Could you check a few things on this drawing? It's one solid part, dimensions in mm from its lowest x, y, z. Give positions to 0.01 mm unless a question says otherwise; leave off trailing zeros. Use one line per item in the form item = value.
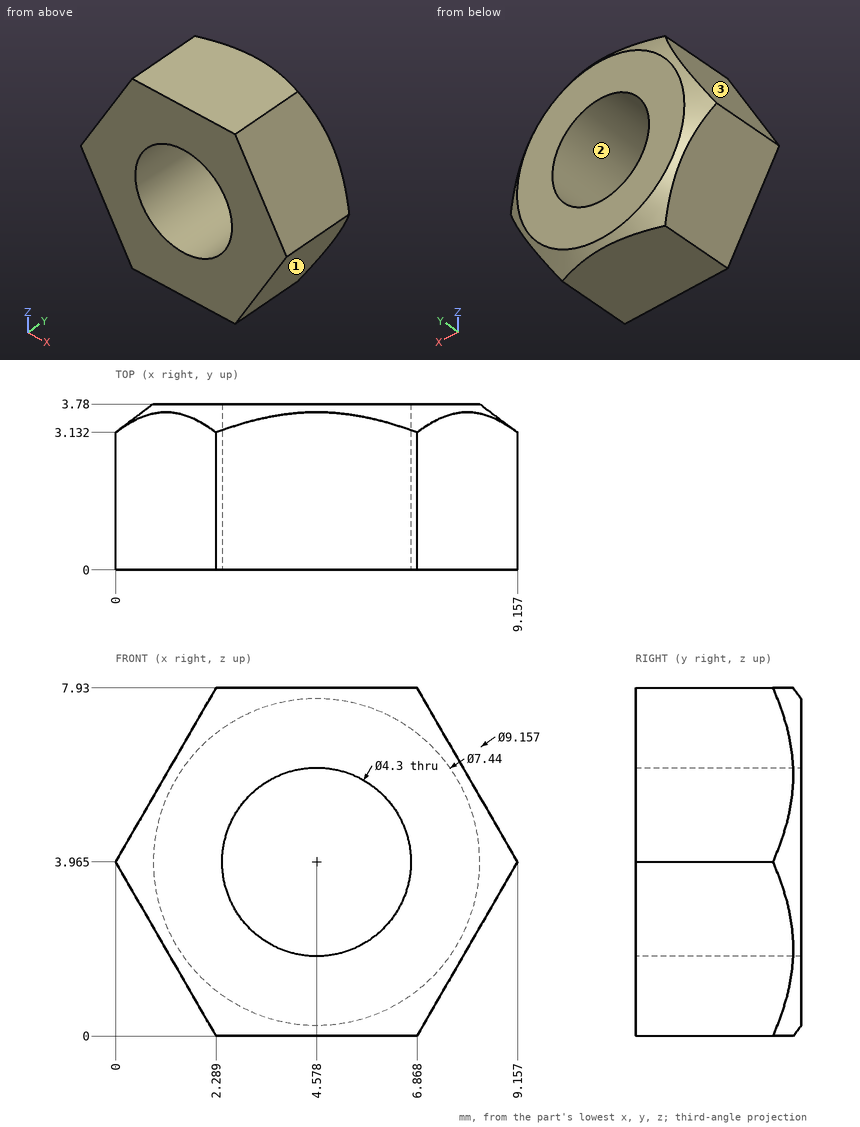
Q1. I need wall thicknesses on L1, parallel to X at y = 2.55, z = 5.5 (1 decimal); L2, parallel to X at y = 1.1, z = 4.75 (1 decimal); L3, parallel to Z at x = 6.5, y = 0.55 (1 decimal). Which ranges of each line are inside material? Lowest first, please.
Found:
L1 = 0.9 to 3.1, 6.1 to 8.3
L2 = 0.5 to 2.6, 6.6 to 8.7
L3 = 0 to 3, 4.9 to 7.9
Q2. Thinking about a two-plate mould opening in X: for the marked faces 1, 2 and 3, which applies, +X half, -X half, draft (parallel to the pull), parting line (faces both ways), or undercut?
Found:
face_1 = +X half
face_2 = undercut
face_3 = -X half
Q3. I'm going to push a flat-ended pin straight in: pin 1 Ø1.5 at (x, y) = (8, 2.5) entering from +Z. Where does the tip first touch, or does it pass through?
Found:
pin_1 = 7.27
